The listing builds one solid part. Answer for the finished solid, in the listing's coordinates (mm). Face numbers are marked on the shaded views. A direction names the side the tool comes from. Coordinates: 2 decimals unless noted, no trailing zeros. Order: outer loops, then holes, each group sorted by start corner. A loop starts at its lowest first (then second) coordinate and runs counter-clockwise, first axis right, second up. Notation, with made-up numbers: (-34.75, -28.5) -> (-29.75, -28.5) arc R9 cw to (-29.75, -16.5) -> close; hole circle Ø3 at (77, 18). An arc over 180 degrees is marked (long way). Answer in a Markdown table with one row per item.
```python
from build123d import *

# Parameters (mm, degrees)
SKETCH1_W           = 14
SKETCH1_H           = 29.7
BOSS_EXTRUDE1_DEPTH = 17
SKETCH2_R           = 2
CUT_EXTRUDE1_DEPTH  = 30.7
SKETCH3_R           = 4
CUT_EXTRUDE2_DEPTH  = 27.7
CUT_EXTRUDE4_START  = -2
SKETCH4_W           = 10
SKETCH4_H           = 13
CUT_EXTRUDE4_DEPTH  = 25.7
BOSS_EXTRUDE2_DEPTH = 1.5


with BuildPart() as part:
    # Sketch1 → Boss-Extrude1 (new body)
    with BuildSketch(Plane.XY):
        with Locations((7, 14.85)):
            Rectangle(SKETCH1_W, SKETCH1_H)
    extrude(amount=BOSS_EXTRUDE1_DEPTH)

    # Sketch2 → Cut-Extrude1 (cut, through all)
    with BuildSketch(Plane(origin=(0, 29.7, 0), x_dir=(1, 0, 0), z_dir=(0, 1, 0))):
        with Locations((7, -8.5)):
            Circle(SKETCH2_R)
    extrude(amount=-CUT_EXTRUDE1_DEPTH, mode=Mode.SUBTRACT)

    # Sketch3 → Cut-Extrude2 (cut)
    with BuildSketch(Plane.XZ):
        with Locations((7, 8.5)):
            Circle(SKETCH3_R)
    extrude(amount=-CUT_EXTRUDE2_DEPTH, mode=Mode.SUBTRACT)

    # Sketch4 → Cut-Extrude4 (cut)
    with BuildSketch(Plane.XZ.offset(CUT_EXTRUDE4_START)):
        with Locations((7, 8.5)):
            Rectangle(SKETCH4_W, SKETCH4_H)
    extrude(amount=-CUT_EXTRUDE4_DEPTH, mode=Mode.SUBTRACT)

    # Sketch5 → Boss-Extrude2 (add)
    with BuildSketch(Plane.XY.offset(17)):
        with BuildLine():
            ThreePointArc((0, 23.1), (-2.1, 21), (-4.2, 23.1))
            Line((-4.2, 23.1), (-4.2, 24.1))
            ThreePointArc((-4.2, 24.1), (-2.1, 26.2), (0, 24.1))
            Line((0, 24.1), (0, 29.7))
            ThreePointArc((0, 29.7), (-0.61507576, 28.21507576), (-2.1, 27.6))
            ThreePointArc((-2.1, 27.6), (-6.1, 23.6), (-2.1, 19.6))
            ThreePointArc((-2.1, 19.6), (-0.61507576, 18.98492424), (0, 17.5))
            Line((0, 17.5), (0, 23.1))
        make_face()
        with BuildLine():
            Line((14, 5.6), (14, 0))
            ThreePointArc((14, 0), (14.61507576, 1.48492424), (16.1, 2.1))
            ThreePointArc((16.1, 2.1), (20.1, 6.1), (16.1, 10.1))
            ThreePointArc((16.1, 10.1), (14.61507576, 10.71507576), (14, 12.2))
            Line((14, 12.2), (14, 6.6))
            ThreePointArc((14, 6.6), (16.1, 8.7), (18.2, 6.6))
            Line((18.2, 6.6), (18.2, 5.6))
            ThreePointArc((18.2, 5.6), (16.1, 3.5), (14, 5.6))
        make_face()
    extrude(amount=-BOSS_EXTRUDE2_DEPTH)


solid = part.part
```
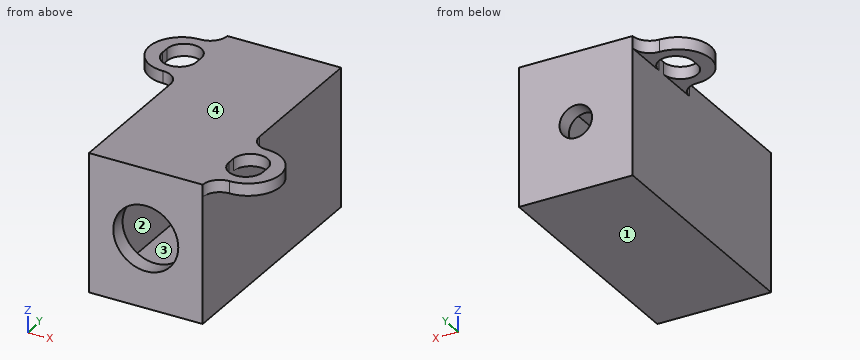
(1) A cutting plane is placed at C-C, the plane x = 7.5. Determine the outline of the cut face in (y, z), then the cut area to 3 significant figures.
Check values:
| item | result |
|---|---|
| outline | (0, 0) -> (29.7, 0) -> (29.7, 6.56) -> (27.7, 6.56) -> (27.7, 2) -> (2, 2) -> (2, 4.53) -> (0, 4.53) -> close; (0, 12.47) -> (2, 12.47) -> (2, 15) -> (27.7, 15) -> (27.7, 10.44) -> (29.7, 10.44) -> (29.7, 17) -> (0, 17) -> close |
| area | 147 mm² |
(2) Which of the six approach directions +Z, -Z, +X, -X, +Y, -Y give full straight-line access (tool end or side, diameter ignored) to the marked faces 1 and 2?
Check values:
| item | result |
|---|---|
| face 1 | -Z, +X, -X, +Y, -Y |
| face 2 | none |
(3) Find the intervals of material crossed by line 1 along Z through (x, y) = (7, 28.9); line 2 along Y through (x, z) = (9.5, 13.25); line 3 along X through (y, z) = (29.2, 8.5), in increasing order. Write a range as from..to.
Check values:
| item | result |
|---|---|
| line 1 | 0..6.5, 10.5..17 |
| line 2 | 0..2, 27.7..29.7 |
| line 3 | 0..5, 9..14 |
(4) A cutting plane is placed at D-D, the plane z = 8.5. Determine the outline of the cut face in (x, y).
Check values:
| item | result |
|---|---|
| outline | (0, 0) -> (3, 0) -> (3, 2) -> (2, 2) -> (2, 27.7) -> (5, 27.7) -> (5, 29.7) -> (0, 29.7) -> close; (9, 27.7) -> (12, 27.7) -> (12, 2) -> (11, 2) -> (11, 0) -> (14, 0) -> (14, 29.7) -> (9, 29.7) -> close |
(5) For a pull along X with two mould halves and no side action, classify the marked faces 3 and 4 as released by +X, released by -X, zero draft, split by the parting line, or undercut.
Check values:
| item | result |
|---|---|
| face 3 | undercut |
| face 4 | zero draft |
(6) A cutting plane is placed at B-B, the plane z = 14. Determine the outline of the cut face in (x, y), then the cut area to 3 significant figures.
Check values:
| item | result |
|---|---|
| outline | (0, 0) -> (14, 0) -> (14, 29.7) -> (0, 29.7) -> close; hole (2, 2) -> (12, 2) -> (12, 27.7) -> (2, 27.7) -> close |
| area | 159 mm² |
(7) A cutting plane is placed at A-A, the plane y = 23.6. Determine the outline of the cut face in (x, z), then the cut area to 3 significant figures.
Check values:
| item | result |
|---|---|
| outline | (-6.1, 15.5) -> (-4.2, 15.5) -> (-4.2, 17) -> (-6.1, 17) -> close; (0, 0) -> (14, 0) -> (14, 17) -> (0, 17) -> close; hole (2, 2) -> (12, 2) -> (12, 15) -> (2, 15) -> close |
| area | 111 mm² |
(8) Flat-ended cylindrical pins translate along their axes: pin 1 (3 mm diameter, centred on x = -4.5, y = 24, fed in from -Z); pin 2 (8.5 mm diameter, centred on y = 9.5, z = 12.5, fed in from -X); pin 3 (0.8 mm diameter, centred on y = 23.5, z = 16, fed in from +X). Find the tip coordinate at first contact, or state that the pin passes through.
Check values:
| item | result |
|---|---|
| pin 1 | z = 15.5 |
| pin 2 | x = 0 |
| pin 3 | x = 14 |
